The model under review builds one solid part; all positions refer to its coordinate system, in mm. A direction names the side the tool comes from. Give positions to 0.01 mm unless a question says otherwise; leave off trailing zeros. Order: outer loops, then holes, each group sorted by start corner. A loop starts at its lowest first (then second) coordinate and runs counter-clockwise, first axis right, second up. Notation, with made-up numbers: M 41,54.5 L 60,54.5 A15 ccw 60,81.5 Z; hole C -17.75,60 d3. An arc over 180 degrees is marked long. One line per question, with ' | ' between items. Start each with the question number.
1. Wall thickness on L1, parallel to X at y = -7.25, z = 1.3; L2, parallel to X at y = -8, z = 1.2; L3, parallel to X at y = -2, z = 2.3: over which ranges is each line inside the solid? List them lowest first.
2. We need section D-D on x = 27.5. Write out the cut boundary in (y, z).
3. Insertion check: P1, Ø2, axis at y = -7, z = 3, coming from the +X side; P2, Ø2, axis at x = 16.5, z = 1, coming from the +Y side; P3, Ø2, axis at y = -5, z = 2, coming from the -X side. Each pin has a flat end and moves straight along its axis. Give the tip position at first contact, or say it passes through.
4. For faces 1 (the face through (19.114, -4.195, 1.972)), 2 (the face through (31.002, -8.944, 1.972)), 3 (the face through (40.7, -7.42, 1.97)), list the 3-axis set-ups (+Z, -Z, +X, -X, +Y, -Y) from which the entire face can be reached by the end or side of a thin tool; tool diameter is ignored.
5. The part is to be moulded in two halves that separate along X. For faces 4 (the face through (28, -8, 0)), 5 (the face through (21.97, -8.91, 1.97)), 6 (the face through (41.318, -14.035, 1.972)), say which applies: +X half, -X half, draft (parallel to the pull), parting line (faces both ways), or undercut.
6. We need section C-C on y = -6. Write out the cut boundary in (x, z).
7. We need section A-A on z = 0.9. Write out the cut boundary in (x, y), then the cut area to 3 significant figures.
8. We need section B-B on x = 45.5. Write out the cut boundary in (y, z).
```python
from build123d import *

# Parameters (mm, degrees)
SKETCH1_R           = 0.75
SKETCH1_R_2         = 1.25
SKETCH1_R_3         = 1
BOSS_EXTRUDE2_DEPTH = 4


with BuildPart() as part:
    # Sketch1 → Boss-Extrude2 (new body)
    with BuildSketch(Plane.XY):
        with BuildLine():
            Line((18.405783089, -9.376058657), (25.628644526, -8.435404146))
            ThreePointArc((25.628644526, -8.435404146), (27.202023368, -8.355640481), (28.768404416, -8.523966464))
            Line((28.768404416, -8.523966464), (33.299022581, -9.376058657))
            Line((33.299022581, -9.376058657), (34.120905067, -11.430554242))
            ThreePointArc((34.120905067, -11.430554242), (41.429155101, -14.002085417), (46.007385343, -7.752037497))
            ThreePointArc((46.007385343, -7.752037497), (48.022828461, -2.701791829), (42.620210155, -2.0863995))
            ThreePointArc((42.620210155, -2.0863995), (37.707004122, -1.546981728), (33.834920639, -4.619038785))
            Line((33.834920639, -4.619038785), (25.885206346, -3.723470434))
            ThreePointArc((25.885206346, -3.723470434), (24.544626829, -3.66305828), (23.20802923, -3.782682405))
            Line((23.20802923, -3.782682405), (14.904254879, -4.619038785))
            ThreePointArc((14.904254879, -4.619038785), (8.82513363, -6.767310768), (13.813095481, -10.852775766))
            Line((13.813095481, -10.852775766), (16.06646506, -9.974716914))
            ThreePointArc((16.06646506, -9.974716914), (17.21798795, -9.604519035), (18.405783089, -9.376058657))
        make_face()
        with Locations((12.469720998, -7.405262894)):
            Circle(SKETCH1_R, mode=Mode.SUBTRACT)
        with Locations((39.507512119, -7.792633892)):
            Circle(SKETCH1_R_2, mode=Mode.SUBTRACT)
        with Locations((45.086512481, -4.457254609)):
            Circle(SKETCH1_R_3, mode=Mode.SUBTRACT)
    extrude(amount=BOSS_EXTRUDE2_DEPTH)


solid = part.part
```
Entries:
1) L1: x = 8.77 to 11.74, 13.2 to 38.38, 40.63 to 47.06 | L2: x = 8.82 to 12.01, 12.93 to 38.27, 40.74 to 46 | L3: x = 36.56 to 42.46, 42.71 to 47.47
2) outline: M -8.37,0 L -3.91,0 L -3.91,4 L -8.37,4 Z
3) P1: stops at x = 48.14 | P2: stops at y = -4.36 | P3: stops at x = 9.05
4) face 1: +Z, -Z, +Y | face 2: +Z, -Z, -Y | face 3: +Z, -Z
5) face 4: draft | face 5: undercut | face 6: parting line
6) outline: M 9.05,0 L 48.14,0 L 48.14,4 L 9.05,4 Z
7) outline: M 13.81,-10.85 L 16.07,-9.97 A10 cw 18.41,-9.38 L 25.63,-8.44 A10 cw 28.77,-8.52 L 33.3,-9.38 L 34.12,-11.43 A6.5 ccw 46.01,-7.75 A3.42 ccw long 42.62,-2.09 A6.5 ccw 33.83,-4.62 L 25.89,-3.72 A10 ccw 23.21,-3.78 L 14.9,-4.62 A3.7 ccw long Z; hole C 12.47,-7.41 d1.5; hole C 39.51,-7.79 d2.5; hole C 45.09,-4.46 d2 | area: 271 mm^2
8) outline: M -10.31,0 L -5.37,0 L -5.37,4 L -10.31,4 Z; M -3.55,0 L -1.06,0 L -1.06,4 L -3.55,4 Z
